Input: part model. Units: mm. Frame: model coordinates. A direction names the side the tool comes from. Round coordinates to 2 decimals unless told otherwise and drop trailing zeros. Loops run counter-clockwise (first coordinate to the right, second up) from the corner with the lowest first, then second, coordinate; pieces in that order, holes last. Notation, with made-up numbers: (15, -8) -> (45, -8) arc R10 ccw to (45, 1) -> close; hole circle Ø11 at (34, 68). An arc over 180 degrees is marked (long way). One line per question, with ' | ' between items. Start each with the question number.
Q1. Material intervals for L1, parallel to Z at x = 0, y = -1.35; L2, parallel to Z at x = -2.25, y = -8.25; L3, parallel to Y at x = 9.75, z = -6.25, sorted ascending.
Q2. Access query for faces 4 (the face through (3, -3.175, -3)), 5 (the face through (1, -10.922, 5)), 6 (the face through (-4.14, -6.57, -9.09)). Directions: +Z, -Z, +X, -X, +Y, -Y. A direction counts if a zero-diameter tool reaches every point of the face in a straight line with its end or side. Return the directions, or none.
Q3. Cut plane C-C on x = 2.75. Return loops of the section in (y, z) (3 decimals).
Q4. Mould query, pull axis X, two halves, no side actions, for faces 1 (the face through (5, 0, 0)), 2 (the face through (-1.38, -10.02, -6.2)), 3 (the face through (-3.397, -6.568, 8.66)). Classes: pulls with the +X half, pulls with the -X half, needs draft (parallel to the pull), parting line crosses it, or undercut.
Q5. Cut plane B-B on z = -5.25. Return loops of the section in (x, y), and give its area (3 significant figures).
Q6. Cut plane D-D on y = -6. Return loops of the section in (x, z) (3 decimals), and give its area (3 significant figures).
Q7. Contact query for flat-ended pins moving along their axis: P1, Ø1, axis at x = -1.5, z = -7.5, coming from the -Y side; P2, Ø8.5, axis at x = 0, z = 0, coming from the +Y side (3 decimals); P3, Ø7.5, axis at x = 0, z = 0, coming from the -Y side; P4, Ø2, axis at x = -4.5, y = -9, coming from the +Z side. Output: stop coordinate, or through.
from build123d import *

# Parameters (mm, degrees)
F0_R     = 12.7
F0_R_2   = 3.9751
F1_DEPTH = 9.144
F2_R     = 6.35
F2_R_2   = 3.9751
F3_DEPTH = 1.778
F4_R     = 4.7625
F4_R_2   = 3.9751
F5_DEPTH = 3.175
F6_R     = 4.7625
F6_R_2   = 3.9751
F7_DEPTH = 3.175
F9_D     = 2.8448
F9_DEPTH = 5.08
F9_TIP   = 0.8546641445


with BuildPart() as f1:
    # F0 (on Front) → F1 (new body)
    with BuildSketch(Plane.XZ):
        Circle(F0_R)
        Circle(F0_R_2, mode=Mode.SUBTRACT)
    extrude(amount=F1_DEPTH)

    # F2 (on face) → F3 (join)
    with BuildSketch(Plane.XZ.offset(9.144)):
        Circle(F2_R)
        Circle(F2_R_2, mode=Mode.SUBTRACT)
    extrude(amount=F3_DEPTH)

    # F4 (on face) → F5 (cut)
    with BuildSketch(Plane.XZ.offset(10.922)):
        Circle(F4_R)
        Circle(F4_R_2, mode=Mode.SUBTRACT)
    extrude(amount=-F5_DEPTH, mode=Mode.SUBTRACT)

    # F6 (on face) → F7 (cut)
    with BuildSketch(Plane(origin=(0, 0, 0), x_dir=(-1, 0, 0), z_dir=(0, 1, 0))):
        Circle(F6_R)
        Circle(F6_R_2, mode=Mode.SUBTRACT)
    extrude(amount=-F7_DEPTH, mode=Mode.SUBTRACT)

    # F9
    with Locations(Plane.XZ.offset(9.144)):
        with Locations((8.89, 0), (-4.445, 7.6989658396), (-4.445, -7.6989658396)):
            Hole(F9_D / 2, depth=F9_DEPTH)
            with Locations((0, 0, -(F9_DEPTH + F9_TIP / 2))):  # 118° drill point
                Cone(0, F9_D / 2, F9_TIP, mode=Mode.SUBTRACT)


solid = f1.part
Results:
1) L1: -12.7 to -4.76, 4.76 to 12.7 | L2: -12.5 to -4.2, 4.2 to 12.5 | L3: -9.14 to 0
2) face 4: +Y | face 5: +Z, -Z, +X, -X, -Y | face 6: -Y
3) outline: (-10.922, -5.724) -> (-9.144, -5.724) -> (-9.144, -12.399) -> (0, -12.399) -> (0, -3.888) -> (-3.175, -3.888) -> (-3.175, -2.87) -> (-7.747, -2.87) -> (-7.747, -3.888) -> (-10.922, -3.888) -> close; (-10.922, 3.888) -> (-7.747, 3.888) -> (-7.747, 2.87) -> (-3.175, 2.87) -> (-3.175, 3.888) -> (0, 3.888) -> (0, 12.399) -> (-9.144, 12.399) -> (-9.144, 5.724) -> (-10.922, 5.724) -> close
4) face 1: needs draft | face 2: parting line crosses it | face 3: undercut
5) outline: (-11.56, -9.14) -> (-3.57, -9.14) -> (-3.57, -10.92) -> (3.57, -10.92) -> (3.57, -9.14) -> (11.56, -9.14) -> (11.56, 0) -> (-11.56, 0) -> close | area: 224 mm^2
6) outline: circle Ø25.4 at (0, 0); hole circle Ø2.845 at (-4.445, -7.699); hole circle Ø2.845 at (-4.445, 7.699); hole circle Ø7.95 at (0, 0); hole circle Ø2.845 at (8.89, 0) | area: 438 mm^2
7) P1: y = -9.14 | P2: y = -3.175 | P3: through | P4: z = 12.21
